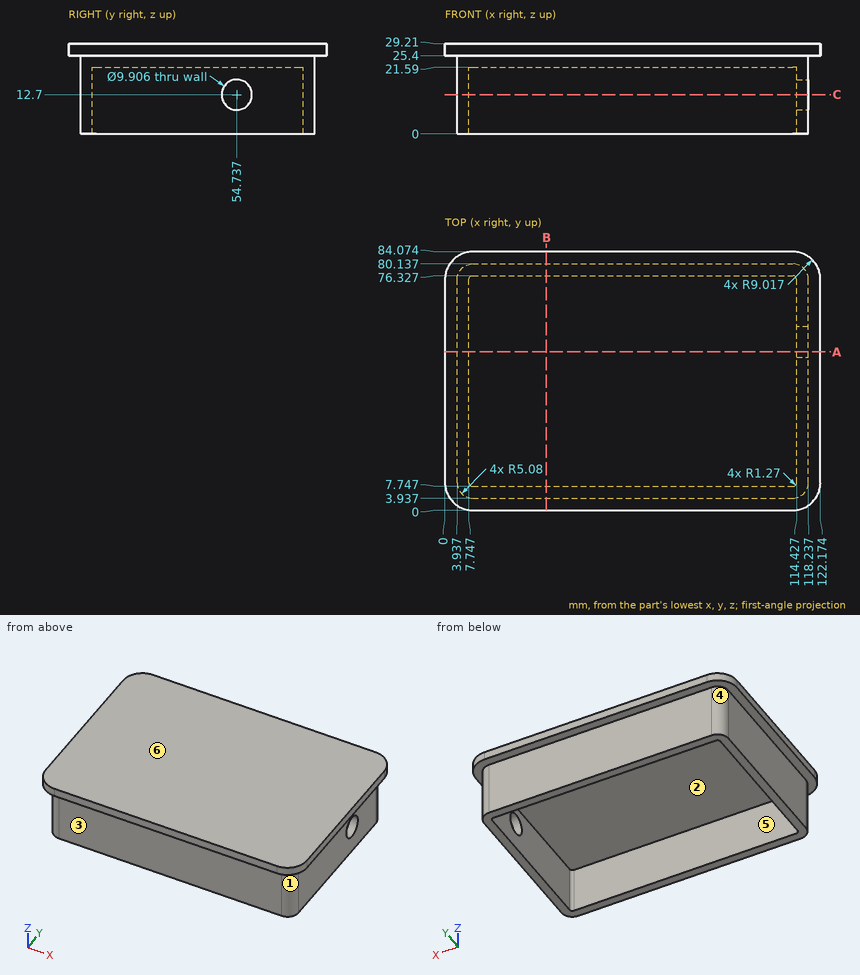
The drawing under review shows one solid part. Ordinate dimensions are in mm from its lowest x, y, z. A direction names the side the tool comes from. Round coordinates to 2 decimals unless told otherwise and drop trailing zeros. Order: outer loops, then holes, each group sorted by start corner. A loop starts at its lowest first (then second) coordinate and runs counter-clockwise, first axis right, second up. Notation, with made-up numbers: (18.25, 27) -> (71.25, 27) arc R25 ccw to (71.25, 39) -> close; hole circle Ø6 at (-29.5, 72). An arc over 180 degrees is marked (long way). Use a Markdown table: item, result.
Item 1: Machinability: for the marked faces 1, 2 and 3, which of the approach directions +Z, -Z, +X, -X, +Y, -Y give a long, thin tool a straight path to every point of the face, cutting with its end or side? Answer none if there is none.
Resolved:
| item | result |
|---|---|
| face 1 | -Z, +X, -Y |
| face 2 | -Z |
| face 3 | -Z, +X, -X, -Y |
Item 2: For line 1 along Y through (x, z) = (94.5, 19.75); line 2 along X through (y, z) = (61.5, 13.5); line 3 along X through (y, z) = (39, 23), list the stretches that pass through material, from the lowest coordinate up. Write a range as [from, to].
Resolved:
| item | result |
|---|---|
| line 1 | y = [3.94, 7.75], [76.33, 80.14] |
| line 2 | x = [3.94, 7.75], [114.43, 118.24] |
| line 3 | x = [3.94, 118.24] |
Item 3: Take a section at B-B (x = 33). State the section outline as (y, z) points.
Resolved:
| item | result |
|---|---|
| outline | (0, 25.4) -> (3.94, 25.4) -> (3.94, 0) -> (7.75, 0) -> (7.75, 21.59) -> (76.33, 21.59) -> (76.33, 0) -> (80.14, 0) -> (80.14, 25.4) -> (84.07, 25.4) -> (84.07, 29.21) -> (0, 29.21) -> close |
Item 4: Draft analysis for pull direction X (two halves, no side actions). For the marked faces 4, 5 and 6, state which applies: +X half, -X half, draft (parallel to the pull), parting line (faces both ways), or undercut.
Resolved:
| item | result |
|---|---|
| face 4 | -X half |
| face 5 | undercut |
| face 6 | draft |
Item 5: Take a section at A-A (y = 51.5). State the section outline as (x, z) points.
Resolved:
| item | result |
|---|---|
| outline | (0, 25.4) -> (3.94, 25.4) -> (3.94, 0) -> (7.75, 0) -> (7.75, 21.59) -> (114.43, 21.59) -> (114.43, 16.45) -> (118.24, 16.45) -> (118.24, 25.4) -> (122.17, 25.4) -> (122.17, 29.21) -> (0, 29.21) -> close; (114.43, 0) -> (118.24, 0) -> (118.24, 8.95) -> (114.43, 8.95) -> close |
Item 6: Take a section at C-C (z = 12.7). State the section outline as (x, y) points, plus the area to 3 significant figures.
Resolved:
| item | result |
|---|---|
| outline | (3.94, 9.02) arc R5.08 ccw to (9.02, 3.94) -> (113.16, 3.94) arc R5.08 ccw to (118.24, 9.02) -> (118.24, 49.78) -> (114.43, 49.78) -> (114.43, 9.02) arc R1.27 cw to (113.16, 7.75) -> (9.02, 7.75) arc R1.27 cw to (7.75, 9.02) -> (7.75, 75.06) arc R1.27 cw to (9.02, 76.33) -> (113.16, 76.33) arc R1.27 cw to (114.43, 75.06) -> (114.43, 59.69) -> (118.24, 59.69) -> (118.24, 75.06) arc R5.08 ccw to (113.16, 80.14) -> (9.02, 80.14) arc R5.08 ccw to (3.94, 75.06) -> close |
| area | 1,340 mm² |
Item 7: For pin 1 (5 mm diameter, centred on x = 19, y = 11.5, fed in from -Z); pin 2 (11 mm diameter, centred on x = 81.5, z = 14, fed in from +Y); pin 3 (17.5 mm diameter, centred on y = 52.5, z = 8, fed in from -X), all flat-tipped, find the tip position at first contact; note any pin that passes through.
Resolved:
| item | result |
|---|---|
| pin 1 | stops at z = 21.59 |
| pin 2 | stops at y = 80.14 |
| pin 3 | stops at x = 3.94 |
